Can you work these out from the model? Positions are in its coordinate system, mm. Face numbers are marked on the shaded views. A direction names the side the tool comes from. Give positions to 0.01 mm unless a question says otherwise; leave off trailing zeros. Write each loop counter-clockwise with the first axis right and the second up, starting at its lowest first coordinate (ties: lowest second). Pieces come first, ordered by that corner, then holes.
from build123d import *

# Parameters (mm, degrees)
F0_W      = 1.5
F0_H      = 12
F2_R      = 6.5
F3_DEPTH  = 25.3
F4_R      = 5.25
F5_DEPTH  = 7.7
F6_R      = 1.6
F7_DEPTH  = 2.3
F8_R      = 4
F9_R      = 0.5
F10_R     = 2.056885
F11_DEPTH = 1


with BuildPart() as f1:
    # F0 (on Front) → F1 (revolve)
    with BuildSketch(Plane.XZ):
        with Locations((-0.75, 2.3)):
            Rectangle(F0_W, F0_H)
    revolve(axis=Axis((0, 0, -10.260424), (0, 0, -1)))

    # F2 (on face) → F3 (join)
    with BuildSketch(Plane.XY.offset(8.3)):
        Circle(F2_R)
    extrude(amount=F3_DEPTH)

    # F4 (on face) → F5 (join)
    with BuildSketch(Plane.XY.offset(33.6)):
        Circle(F4_R)
    extrude(amount=F5_DEPTH)

    # F6 (on face) → F7 (join)
    with BuildSketch(Plane.XY.offset(41.3)):
        with BuildLine():
            Line((-1.494822, 5.994148), (-9.967878, 3.881135))
            ThreePointArc((-9.967878, 3.881135), (-13, 0), (-9.967878, -3.881135))
            Line((-9.967878, -3.881135), (-1.494822, -5.994148))
            ThreePointArc((-1.494822, -5.994148), (0, -6.177726), (1.494822, -5.994148))
            Line((1.494822, -5.994148), (9.967878, -3.881135))
            ThreePointArc((9.967878, -3.881135), (13, 0), (9.967878, 3.881135))
            Line((9.967878, 3.881135), (1.494822, 5.994148))
            ThreePointArc((1.494822, 5.994148), (0, 6.177726), (-1.494822, 5.994148))
        make_face()
        with Locations((-9, 0)):
            Circle(F6_R, mode=Mode.SUBTRACT)
        with Locations((9, 0)):
            Circle(F6_R, mode=Mode.SUBTRACT)
    extrude(amount=F7_DEPTH)

    # F8
    f8_edges = [f1.edges().sort_by_distance(p)[0] for p in [
        (-6.5, 0, 8.3),
    ]]
    fillet(f8_edges, radius=F8_R)

    # F9
    f9_edges = [f1.edges().sort_by_distance(p)[0] for p in [
        (1.5, 0, -3.7),
    ]]
    fillet(f9_edges, radius=F9_R)

    # F10 (on Top) → F11 (join)
    with BuildSketch(Plane.XY):
        Circle(F10_R)
    extrude(amount=F11_DEPTH)


solid = f1.part
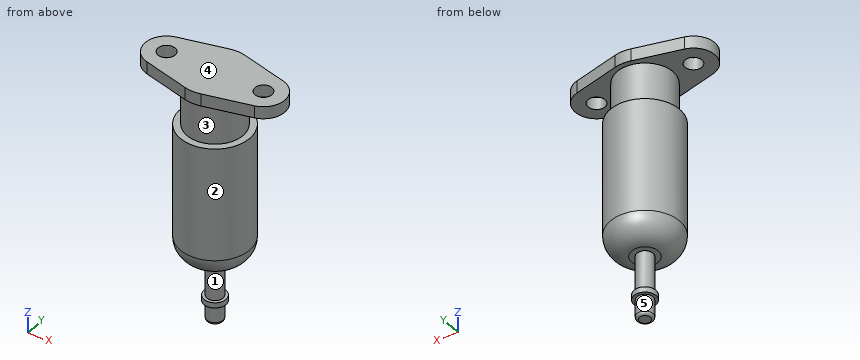
(1) For the marked faces 1 and 2, which set-ups out of +Z, -Z, +X, -X, +Y, -Y let a thin tool reach every point of the face, with its end or its side?
Returned:
face 1: none
face 2: -Z
(2) If we mould it in two halves opening along Z, with no side actions, what happens to the marked faces 3, 4 and 5? For each: +Z half, -Z half, draft (parallel to the pull), parting line (faces both ways), or undercut.
Returned:
face 3: undercut
face 4: +Z half
face 5: draft
(3) Imagine slicing it at B-B, the plane z = 21. Write out the boundary of the cut face in (x, y), plus the area to 3 significant figures.
Returned:
outline: circle Ø13 at (0, 0)
area: 133 mm2
(4) Imagine slicing it at A-A, the plane x = 9. Write out the boundary of the cut face in (y, z).
Returned:
outline: (-4.12, 41.3) - (-1.6, 41.3) - (-1.6, 43.6) - (-4.12, 43.6) - close; (1.6, 41.3) - (4.12, 41.3) - (4.12, 43.6) - (1.6, 43.6) - close
(5) Will these pins go through, and if not, where does the flat tip stop? P1, Ø2, axis at x = 6, y = 2, coming from the -Z side; P2, Ø1, axis at x = 5.5, z = 29.5, coming from the +Y side; P3, Ø2, axis at y = -1, z = 35.5, coming from the +X side.
Returned:
P1: stops at z = 9.47
P2: stops at y = 4.15
P3: stops at x = 5.25
(6) If I drill on L1, parallel to Y at x = 9, z = 42.4; L2, parallel to Z at x = 5.25, y = 2.5; L3, parallel to Z at x = -10.5, y = -2.25, over which ranges is the centre line in solid material (lowest first)?
Returned:
L1: y = -4.12 to -1.6, 1.6 to 4.12
L2: z = 10.06 to 33.6, 41.3 to 43.6
L3: z = 41.3 to 43.6
